Can you work these out from the model? Positions are in its coordinate system, mm. Give positions to 0.01 mm unless a question says otherwise; leave off trailing zeros. Order: outer loops, then holes, each group sorted by start corner. A loop starts at its lowest first (then second) coordinate and runs counter-clockwise, first axis right, second up. Notation, with made-up numbers: (-27.5, 77) - (-8.5, 77) arc R11 ccw to (-8.5, 93) - close; hole circle Ø6 at (-14.5, -27). An arc over 180 degrees is marked (long way). Write each question's results on one line, items separated by ' | '. Start each with the question number.
from build123d import *

# Parameters (mm, degrees)
F0_W     = 90
F0_H     = 95
F0_R     = 1.65
F0_R_2   = 5
F0_W_2   = 80
F0_H_2   = 52
F1_DEPTH = 0.8


with BuildPart() as f1:
    # F0 (on Top) → F1 (new body)
    with BuildSketch(Plane.XY):
        with Locations((45, 47.5)):
            Rectangle(F0_W, F0_H)
        with Locations((3.3, 26.7)):
            Circle(F0_R, mode=Mode.SUBTRACT)
        with Locations((81.25, 16.25)):
            Circle(F0_R_2, mode=Mode.SUBTRACT)
        with Locations((86.7, 26.7)):
            Circle(F0_R, mode=Mode.SUBTRACT)
        with Locations((3.3, 91.7)):
            Circle(F0_R, mode=Mode.SUBTRACT)
        with Locations((45, 59.25)):
            Rectangle(F0_W_2, F0_H_2, mode=Mode.SUBTRACT)
        with Locations((86.7, 91.7)):
            Circle(F0_R, mode=Mode.SUBTRACT)
    extrude(amount=F1_DEPTH)


solid = f1.part
Q1. Will this pin go through, and if not, where does the flat tip stop? P1, Ø3, axis at x = 3.3, y = 91.7, coming from the -Z side.
Q2. If we section it at D-D (y = 26.7): Please give me the cut outline in (x, z), plus the area to 3 significant figures.
Q3. If we section it at B-B (y = 16.25): Please give me the cut outline in (x, z).
Q4. If we section it at A-A (x = 3.3): Please give me the cut outline in (y, z).
Q5. If we section it at C-C (x = 73): Please give me the cut outline in (y, z), plus the area to 3 significant figures.
Q6. Thinking about a two-plate mould opening in Y: for faces 1 (the cylindrical face through (2.9, 25.1, 0.4)), 2 (the flat face through (34, 27, 0.8)), which applies, released by +Y, released by -Y, zero draft, split by the parting line, or undercut?
Q7. If I drill on probe 1 along Y at (x, z) = (3.3, 0.55); probe 2 along Y at (x, z) = (6, 0.35); probe 3 along X at (y, z) = (83.5, 0.35), over which ranges is the centre line in solid material (lowest first)? Write a range as from..to.
Findings below:
1) P1: passes through
2) outline: (0, 0) - (1.65, 0) - (1.65, 0.8) - (0, 0.8) - close; (4.95, 0) - (85.05, 0) - (85.05, 0.8) - (4.95, 0.8) - close; (88.35, 0) - (90, 0) - (90, 0.8) - (88.35, 0.8) - close | area: 66.7 mm2
3) outline: (0, 0) - (76.25, 0) - (76.25, 0.8) - (0, 0.8) - close; (86.25, 0) - (90, 0) - (90, 0.8) - (86.25, 0.8) - close
4) outline: (0, 0) - (25.05, 0) - (25.05, 0.8) - (0, 0.8) - close; (28.35, 0) - (90.05, 0) - (90.05, 0.8) - (28.35, 0.8) - close; (93.35, 0) - (95, 0) - (95, 0.8) - (93.35, 0.8) - close
5) outline: (0, 0) - (33.25, 0) - (33.25, 0.8) - (0, 0.8) - close; (85.25, 0) - (95, 0) - (95, 0.8) - (85.25, 0.8) - close | area: 34.4 mm2
6) face 1: undercut | face 2: zero draft
7) probe 1: y = 0..25.05, 28.35..90.05, 93.35..95 | probe 2: y = 0..33.25, 85.25..95 | probe 3: x = 0..5, 85..90
